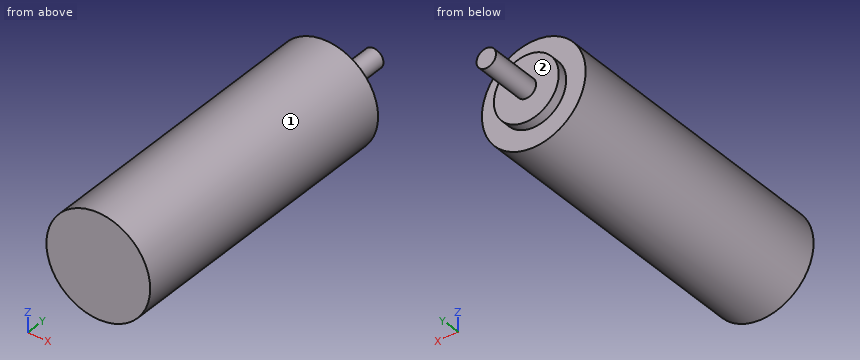
from build123d import *

# Parameters (mm, degrees)
F0_R     = 10
F3_DEPTH = 3
F2_R     = 3
F4_DEPTH = 19.2
F1_R     = 16
F5_DEPTH = 92.1


with BuildPart() as f3:
    # F0 (on Front) → F3 (new body)
    with BuildSketch(Plane.XZ):
        Circle(F0_R)
    extrude(amount=-F3_DEPTH)

    # F2 (on Front) → F4 (join)
    with BuildSketch(Plane.XZ):
        Circle(F2_R)
    extrude(amount=-F4_DEPTH)

    # F1 (on Front) → F5 (join)
    with BuildSketch(Plane.XZ):
        Circle(F1_R)
    extrude(amount=F5_DEPTH)


solid = f3.part
Source: CAD feature listing. Evaluate the final solid. Frame: model axes, mm. Face numbers are marked on the shaded views. A direction names the side the tool comes from. Give positions to 0.01 mm unless a question says otherwise; leave off trailing zeros. Write each loop counter-clockwise with the first axis right and the second up, starting at its lowest first coordinate (ties: lowest second). Pieces come first, ordered by that corner, then holes. Notation, with made-up numbers: M 49,46 L 92,46 A24 ccw 92,78 Z; hole C 27.5,23.25 d7. An arc over 180 degrees is marked long. Return JSON: item names as keys, results as strings. Group by question number.
1) First-contact query: pin 1 Ø6 at (x, z) = (-5, 4.5) entering from +Y; pin 2 Ø10 at (x, y) = (-8, -22.5) entering from +Z; pin 3 Ø6 at (x, y) = (12, -13.5) entering from +Z. Flat tips, straight axial feed; report the tip coordinate or a pass-through.
2) Cut plane C-C, the plane y = -42.5. Output: boundary loops of the cut face in (x, z), then the cut area to 3 significant figures.
3) Cut plane B-B, the plane x = 0. Output: boundary loops of the cut face in (y, z).
4) Cut plane A-A, the plane z = 0. Output: boundary loops of the cut face in (x, y).
5) Ray query, L1, parallel to Y at x = -2, z = -13.5; L2, parallel to Y at x = 5, z = 7; L3, parallel to Z at x = -4.5, y = -39. Return the intervals inside material, ascending.
6) Set-up query: the marked faces 1 and 2. Return all of +Z, -Z, +X, -X, +Y, -Y with unobstructed straight access to the full face (end or side cutting, diameter ignored); none if empty.
7) Cut plane D-D, the plane x = -8. Output: boundary loops of the cut face in (y, z), then the cut area to 3 significant figures.
Data:
{
 "1": {"pin 1": "stops at y = 3", "pin 2": "stops at z = 15.72", "pin 3": "stops at z = 13.23"},
 "2": {"outline": "C 0,0 d32", "area": "804 mm²"},
 "3": {"outline": "M -92.1,-16 L 0,-16 L 0,-10 L 3,-10 L 3,-3 L 19.2,-3 L 19.2,3 L 3,3 L 3,10 L 0,10 L 0,16 L -92.1,16 Z"},
 "4": {"outline": "M -16,-92.1 L 16,-92.1 L 16,0 L 10,0 L 10,3 L 3,3 L 3,19.2 L -3,19.2 L -3,3 L -10,3 L -10,0 L -16,0 Z"},
 "5": {"L1": "y = -92.1 to 0", "L2": "y = -92.1 to 3", "L3": "z = -15.35 to 15.35"},
 "6": {"face 1": "+Y, -Y", "face 2": "+Y"},
 "7": {"outline": "M -92.1,-13.86 L 0,-13.86 L 0,-6 L 3,-6 L 3,6 L 0,6 L 0,13.86 L -92.1,13.86 Z", "area": "2,590 mm²"}
}
